Can you work these out from the model? Positions are in its coordinate system, mm. Round coordinates to 2 decimals unless told otherwise and drop trailing zeros. Loops run counter-clockwise (first coordinate to the right, second up) from the corner with the lowest first, then second, coordinate; pieces in that order, holes last. Notation, with made-up numbers: (12.25, 56.5) -> (56.25, 56.5) arc R33 cw to (56.25, 84.5) -> close; hole circle Ø1 at (3, 85). An arc over 180 degrees is marked (long way). Write each question's results on one line, items separated by ' | '.
from build123d import *

# Parameters (mm, degrees)
BOSS_EXTRUDE1_DEPTH = 2.5
SKETCH2_R           = 0.2
SKETCH2_R_2         = 0.171619636
BOSS_EXTRUDE2_DEPTH = 3.2


with BuildPart() as part:
    # Sketch1 → Boss-Extrude1 (new body)
    with BuildSketch(Plane.XY):
        with BuildLine():
            Line((-2.94, 0), (2.94, 0))
            ThreePointArc((2.94, 0), (0, 2.94), (-2.94, 0))
        make_face()
    extrude(amount=BOSS_EXTRUDE1_DEPTH)

    # Sketch2 → Boss-Extrude2 (add)
    with BuildSketch(Plane.XZ):
        with Locations((-2.54, 1.25)):
            Circle(SKETCH2_R)
        with Locations((2.54, 1.25)):
            Circle(SKETCH2_R_2)
    extrude(amount=BOSS_EXTRUDE2_DEPTH)


solid = part.part
1. If we section it at D-D (z = 2.05): List the corners of the cut face in (x, y) for me, then the cut area to 3 significant figures.
Final values:
outline: (-2.94, 0) -> (2.94, 0) arc R2.94 ccw to start | area: 13.6 mm2
2. Will these pins go through, and if not, where does the flat tip stop? pin 1 (1.2 mm diameter, centred on x = 1, z = 1.5, fed in from -Y); pin 2 (1 mm diameter, centred on x = -2.5, z = 1.5, fed in from +Y).
Final values:
pin 1: y = 0 | pin 2: y = 2.15
3. If we section it at A-A (z = 1.25): List the corners of the cut face in (x, y) for me, then the cut area to 3 significant figures.
Final values:
outline: (-2.94, 0) -> (-2.74, 0) -> (-2.74, -3.2) -> (-2.34, -3.2) -> (-2.34, 0) -> (2.37, 0) -> (2.37, -3.2) -> (2.71, -3.2) -> (2.71, 0) -> (2.94, 0) arc R2.94 ccw to start | area: 16.0 mm2
4. If we section it at C-C (x = 2.5): List the corners of the cut face in (y, z) for me.
Final values:
outline: (-3.2, 1.08) -> (0, 1.08) -> (0, 0) -> (1.55, 0) -> (1.55, 2.5) -> (0, 2.5) -> (0, 1.42) -> (-3.2, 1.42) -> close
5. Please list where these lines run through material, in increasing order: line 1 (Y direction, x = 0, z = 0.3); line 2 (Z direction, x = -2.55, y = -2.75); line 3 (Y direction, x = -2.4, z = 0.6). Write a range as from..to.
Final values:
line 1: 0..2.94 | line 2: 1.05..1.45 | line 3: 0..1.7
6. If we section it at B-B (y = -0.5): List the corners of the cut face in (x, z) for me.
Final values:
outline: circle Ø0.4 at (-2.54, 1.25); circle Ø0.34 at (2.54, 1.25)
